Check sheet for the modelled part. Datum: model origin and axes. Units: mm. Give positions to 0.01 mm unless a question says otherwise; leave off trailing zeros. Loops run counter-clockwise (first coordinate to the right, second up) from the corner with the lowest first, then second, coordinate; pieces in that order, holes last.
```python
from build123d import *


with BuildPart() as f1:
    # F0 (on Front) → F1 (revolve)
    with BuildSketch(Plane.XZ):
        with BuildLine():
            Line((0, 52.7323525879), (0, 40.875408378))
            ThreePointArc((0, 40.875408378), (2.5428559752, 41.4484472615), (4.5941332355, 43.0567854329))
            ThreePointArc((4.5941332355, 43.0567854329), (5.2714168977, 44.0911428638), (5.7194354013, 45.2434830368))
            Line((5.7194354013, 45.2434830368), (5.7194354013, 48.3642779291))
            ThreePointArc((5.7194354013, 48.3642779291), (3.5983335565, 51.5154383055), (0, 52.7323525879))
        make_face()
        with BuildLine():
            ThreePointArc((4.5941332355, 43.0567854329), (2.5428559752, 41.4484472615), (0, 40.875408378))
            Line((0, 40.875408378), (0, -45.7190386951))
            Line((0, -45.7190386951), (3.4478881862, -45.7190386951))
            Line((3.4478881862, -45.7190386951), (3.4478881862, -19.2569392537))
            add(Edge.make_bspline(
                [(3.4478881862, -13.3570219138), (2.8592867201, -14.6215324154), (1.6885418308, -17.0881375195), (2.8291799419, -18.4821080295), (3.4478881862, -19.2569392537)],
                knots=[0.688463947, 0.688463947, 0.688463947, 0.688463947, 0.7466101854, 0.8030070578, 0.8030070578, 0.8030070578, 0.8030070578], degree=3))
            Line((3.4478881862, -13.3570219138), (3.4478881862, -7.214912314))
            add(Edge.make_bspline(
                [(3.4478881862, -2.8591748229), (3.0716325194, -3.8760817958), (2.5489190603, -5.5383480748), (3.1511995592, -6.7331145443), (3.4478881862, -7.214912314)],
                knots=[0.4920828694, 0.4920828694, 0.4920828694, 0.4920828694, 0.5392256635, 0.5731916963, 0.5731916963, 0.5731916963, 0.5731916963], degree=3))
            Line((3.4478881862, -2.8591748229), (3.4478881862, 4.3427177675))
            add(Edge.make_bspline(
                [(3.4478881862, 10.5023898497), (2.8570440893, 9.3644165827), (1.6733580005, 7.094819903), (2.8612423375, 5.2737567308), (3.4478881862, 4.3427177675)],
                knots=[0.2610073473, 0.2610073473, 0.2610073473, 0.2610073473, 0.3169983169, 0.372231172, 0.372231172, 0.372231172, 0.372231172], degree=3))
            Line((3.4478881862, 10.5023898497), (3.4478881862, 16.2601063118))
            add(Edge.make_bspline(
                [(3.4478881862, 22.269270102), (2.5941060701, 21.0188723902), (1.3322312845, 18.8748269949), (2.8529664918, 17.0479984025), (3.4478881862, 16.2601063118)],
                knots=[0.0322061563, 0.0322061563, 0.0322061563, 0.0322061563, 0.1038810888, 0.1549480731, 0.1549480731, 0.1549480731, 0.1549480731], degree=3))
            add(Edge.make_bspline(
                [(4.5941332355, 23.9438803276), (4.2387639607, 23.3926426614), (3.8315235702, 22.8311193108), (3.4478881862, 22.269270102)],
                knots=[0, 0, 0, 0, 0.0322061563, 0.0322061563, 0.0322061563, 0.0322061563], degree=3))
            Line((4.5941332355, 23.9438803276), (4.5941332355, 43.0567854329))
        make_face()
        with BuildLine():
            Line((3.4478881862, -19.2569392537), (3.4478881862, -45.7190386951))
            Line((3.4478881862, -45.7190386951), (4.5941332355, -45.7190386951))
            Line((4.5941332355, -45.7190386951), (4.5941332355, -34.9797420204))
            add(Edge.make_bspline(
                [(3.4478881862, -19.2569392537), (3.8524540819, -19.7635920922), (6.1440033012, -22.672173393), (5.1174351412, -29.440924003), (4.5941332355, -34.9797420204)],
                knots=[0.8030070578, 0.8030070578, 0.8030070578, 0.8030070578, 0.8398842958, 1, 1, 1, 1], degree=3))
        make_face()
        with BuildLine():
            Line((3.4478881862, 22.1658609807), (3.4478881862, 22.269270102))
            add(Edge.make_bspline(
                [(3.4478881862, 22.269270102), (2.5941060701, 21.0188723902), (1.3322312845, 18.8748269949), (2.8529664918, 17.0479984025), (3.4478881862, 16.2601063118)],
                knots=[0.0322061563, 0.0322061563, 0.0322061563, 0.0322061563, 0.1038810888, 0.1549480731, 0.1549480731, 0.1549480731, 0.1549480731], degree=3))
            Line((3.4478881862, 16.2601063118), (3.4478881862, 22.1658609807))
        make_face()
        with BuildLine():
            add(Edge.make_bspline(
                [(3.4478881862, -13.3570219138), (2.8592867201, -14.6215324154), (1.6885418308, -17.0881375195), (2.8291799419, -18.4821080295), (3.4478881862, -19.2569392537)],
                knots=[0.688463947, 0.688463947, 0.688463947, 0.688463947, 0.7466101854, 0.8030070578, 0.8030070578, 0.8030070578, 0.8030070578], degree=3))
            Line((3.4478881862, -19.2569392537), (3.4478881862, -13.3570219138))
        make_face()
        with BuildLine():
            add(Edge.make_bspline(
                [(3.4478881862, 16.2601063118), (4.0076291368, 15.5188062853), (5.1693722085, 13.8280653656), (4.0600606664, 11.6814418551), (3.4478881862, 10.5023898497)],
                knots=[0.1549480731, 0.1549480731, 0.1549480731, 0.1549480731, 0.2029952069, 0.2610073473, 0.2610073473, 0.2610073473, 0.2610073473], degree=3))
            Line((3.4478881862, 16.2601063118), (3.4478881862, 10.5023898497))
        make_face()
        with BuildLine():
            Line((3.4478881862, -7.214912314), (3.4478881862, -13.3570219138))
            add(Edge.make_bspline(
                [(3.4478881862, -7.214912314), (3.9409970185, -8.0156802369), (5.1987251645, -9.5462290276), (4.0433028257, -12.0778744637), (3.4478881862, -13.3570219138)],
                knots=[0.5731916963, 0.5731916963, 0.5731916963, 0.5731916963, 0.6296446549, 0.688463947, 0.688463947, 0.688463947, 0.688463947], degree=3))
        make_face()
        with BuildLine():
            Line((3.4478881862, 4.3427177675), (3.4478881862, 10.5023898497))
            add(Edge.make_bspline(
                [(3.4478881862, 10.5023898497), (2.8570440893, 9.3644165827), (1.6733580005, 7.094819903), (2.8612423375, 5.2737567308), (3.4478881862, 4.3427177675)],
                knots=[0.2610073473, 0.2610073473, 0.2610073473, 0.2610073473, 0.3169983169, 0.372231172, 0.372231172, 0.372231172, 0.372231172], degree=3))
        make_face()
        with BuildLine():
            add(Edge.make_bspline(
                [(3.4478881862, -2.8591748229), (3.0716325194, -3.8760817958), (2.5489190603, -5.5383480748), (3.1511995592, -6.7331145443), (3.4478881862, -7.214912314)],
                knots=[0.4920828694, 0.4920828694, 0.4920828694, 0.4920828694, 0.5392256635, 0.5731916963, 0.5731916963, 0.5731916963, 0.5731916963], degree=3))
            Line((3.4478881862, -7.214912314), (3.4478881862, -2.8591748229))
        make_face()
        with BuildLine():
            add(Edge.make_bspline(
                [(3.4478881862, 4.3427177675), (3.9738604296, 3.5079711254), (5.2405247997, 1.4357055196), (4.0092155805, -1.342074107), (3.4478881862, -2.8591748229)],
                knots=[0.372231172, 0.372231172, 0.372231172, 0.372231172, 0.4217515918, 0.4920828694, 0.4920828694, 0.4920828694, 0.4920828694], degree=3))
            Line((3.4478881862, 4.3427177675), (3.4478881862, -2.8591748229))
        make_face()
    revolve(axis=Axis((0, 0, -2.4218151586), (0, 0, 1)))

    # F2 (on Front) → F3 (revolve)
    with BuildSketch(Plane.XZ):
        with BuildLine():
            Line((19.0536882728, -41.1168672144), (0, -41.1168672144))
            Line((0, -41.1168672144), (0, -53.5302367061))
            Line((0, -53.5302367061), (27.9317204824, -53.5302367061))
            ThreePointArc((27.9317204824, -53.5302367061), (26.9548916276, -47.0361865237), (24.1108555347, -41.1168672144))
            Line((24.1108555347, -41.1168672144), (21.6025765985, -42.9510511458))
            Line((21.6025765985, -42.9510511458), (19.0536882728, -41.1168672144))
        make_face()
        with BuildLine():
            Line((0, -53.5302367061), (0, -41.1168672144))
            Line((0, -41.1168672144), (-19.0536882728, -41.1168672144))
            Line((-19.0536882728, -41.1168672144), (-21.6025765985, -42.9510511458))
            Line((-21.6025765985, -42.9510511458), (-24.1108555347, -41.1168672144))
            ThreePointArc((-24.1108555347, -41.1168672144), (-26.9548916276, -47.0361865237), (-27.9317204824, -53.5302367061))
            Line((-27.9317204824, -53.5302367061), (0, -53.5302367061))
        make_face()
    revolve(axis=Axis((-13.9658602412, 0, -53.5302367061), (1, 0, 0)))


solid = f1.part
```
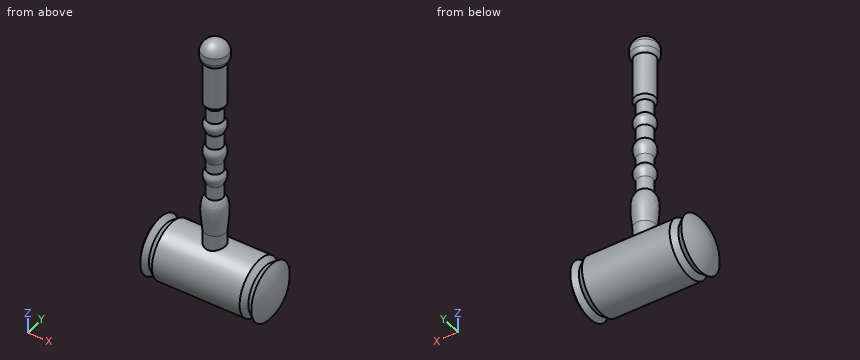
(1) Section check B-B on x = -13.5. Record the boundary of the cut face in (y, z), plus the area to 3 significant figures.
(2) Material ranges on line 1 (X direction, y = 10.75, z = -56); line 2 (Y direction, x = 0, z = -35); line 3 (X direction, y = 0.5, z = -54), recorded low to high.
(3) Gauge pin test, flat ends, axial feed: pin 1 Ø12 at (y, z) = (-6.5, -21) entering from -X; pin 2 Ø4 at (y, z) = (-4.5, -17) entering from +X; pin 3 Ø1 at (x, y) = (-6.5, 8.5) entering from -Z. Record the tip position at first contact, or that the pin passes through.
(4) Section check A-A on z = 30. Record the boundary of the cut face in (x, y).
Computed values:
1. outline: circle Ø24.83 at (0, -53.53)
1. area: 484 mm2
2. line 1: x = -24.98 to -22.22, -20.98 to 20.98, 22.22 to 24.98
2. line 2: y = -4.59 to 4.59
2. line 3: x = -27.92 to 27.92
3. pin 1: stops at x = -5.12
3. pin 2: stops at x = 2.37
3. pin 3: stops at z = -63.02
4. outline: circle Ø9.19 at (0, 0)
